from build123d import *

# Parameters (mm, degrees)
F0_R     = 2.54
F1_DEPTH = 3.96875
F2_W     = 1.6891
F2_H     = 1.56845
F2_W_2   = 1.56845
F2_H_2   = 1.6891
F3_DEPTH = 11.90625


with BuildPart() as f1:
    # F0 (on Top) → F1 (new body, symmetric)
    with BuildSketch(Plane.XY):
        Circle(F0_R)
    extrude(amount=F1_DEPTH, both=True)

    # F2 (on Top) → F3 (join, symmetric)
    with BuildSketch(Plane.XY):
        with Locations((0, 1.628775)):
            Rectangle(F2_W, F2_H)
        with Locations((1.628775, 0)):
            Rectangle(F2_W_2, F2_H_2)
        Rectangle(F2_W, F2_H_2)
        with Locations((-1.628775, 0)):
            Rectangle(F2_W_2, F2_H_2)
        with Locations((0, -1.628775)):
            Rectangle(F2_W, F2_H)
    extrude(amount=F3_DEPTH, both=True)


solid = f1.part
The listing builds one solid part. Answer for the finished solid, in the listing's coordinates (mm). A direction names the side the tool comes from. Coordinates: 2 decimals unless noted, no trailing zeros. Write each loop counter-clockwise with the first axis right and the second up, starting at its lowest first coordinate (ties: lowest second). Pieces come first, ordered by that corner, then holes. Notation, with made-up numbers: (-4, 41) - (38, 41) arc R19 cw to (38, 58) - close; hole circle Ø3 at (53.5, -7.75). An arc over 180 degrees is marked (long way). Return JSON: item names as keys, results as strings.
1. Which of the six approach directions +Z, -Z, +X, -X, +Y, -Y give full straight-line access (tool end or side, diameter ignored) to faces 1 (the face through (-2, -0.845, 5)), 2 (the face through (0.845, 2, 5)), 3 (the face through (0.845, -2, 5))?
Final values:
{"face 1": "-X, -Y", "face 2": "+X, +Y", "face 3": "+X, -Y"}
2. Each of these flat-tipped pins is pushed along its axis until it touches: pin 1 Ø2 at (x, z) = (-2, 9.5) entering from -Y; pin 2 Ø0.8 at (x, y) = (-2, -1.5) entering from +Z; pin 3 Ø2 at (x, y) = (2, 2) entering from -Z. Where does it stop, or does it pass through?
Final values:
{"pin 1": "y = -0.84", "pin 2": "z = 3.97", "pin 3": "z = -3.97"}
3. The part is cut by section A-A on z = -9.75. Determine the outline of the cut face in (x, y).
Final values:
{"outline": "(-2.41, -0.84) - (-0.84, -0.84) - (-0.84, -2.41) - (0.84, -2.41) - (0.84, -0.84) - (2.41, -0.84) - (2.41, 0.84) - (0.84, 0.84) - (0.84, 2.41) - (-0.84, 2.41) - (-0.84, 0.84) - (-2.41, 0.84) - close"}
4. Consider line 1 along Y through (x, z) = (-0.05, -5.25); line 2 along Y through (x, z) = (-1.4, 7). Determine where each line is inside the solid, lowest interval first.
Final values:
{"line 1": "-2.41 to 2.41", "line 2": "-0.84 to 0.84"}
5. The part is cut by section B-B on x = 0.35. Determine the outline of the cut face in (y, z).
Final values:
{"outline": "(-2.52, -3.97) - (-2.41, -3.97) - (-2.41, -11.91) - (2.41, -11.91) - (2.41, -3.97) - (2.52, -3.97) - (2.52, 3.97) - (2.41, 3.97) - (2.41, 11.91) - (-2.41, 11.91) - (-2.41, 3.97) - (-2.52, 3.97) - close"}
